from build123d import *

# Parameters (mm, degrees)
F0_W     = 25
F0_H     = 20
F1_DEPTH = 1
F3_DEPTH = 8


with BuildPart() as f1:
    # F0 (on Top) → F1 (new body)
    with BuildSketch(Plane.XY):
        Rectangle(F0_W, F0_H)
    extrude(amount=F1_DEPTH)

    # F2 (on Front) → F3 (join, symmetric)
    with BuildSketch(Plane.XZ):
        with BuildLine():
            Line((8.940514, 3.397746), (1.101284, 7.244365))
            ThreePointArc((1.101284, 7.244365), (0, 7.5), (-1.101284, 7.244365))
            Line((-1.101284, 7.244365), (-8.940514, 3.397746))
            ThreePointArc((-8.940514, 3.397746), (-9.348679, 3.028908), (-9.5, 2.5))
            Line((-9.5, 2.5), (-9.5, 0.999067))
            Line((-9.5, 0.999067), (9.5, 0.999067))
            Line((9.5, 0.999067), (9.5, 2.5))
            ThreePointArc((9.5, 2.5), (9.348679, 3.028908), (8.940514, 3.397746))
        make_face()
    extrude(amount=F3_DEPTH, both=True)


solid = f1.part
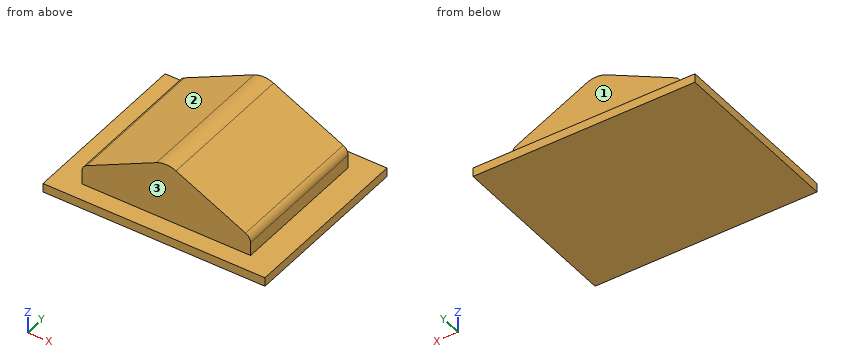
Could you check a few things on this model? Use its own coordinates, in mm. Face numbers are marked on the shaded views. A direction names the side the tool comes from. Give positions to 0.01 mm unless a question says otherwise; leave off trailing zeros. Order: outer loops, then holes, each group sorted by start corner. A loop starts at its lowest first (then second) coordinate and runs counter-clockwise, first axis right, second up. Notation, with made-up numbers: (55.5, -21) - (111.5, -21) arc R13 ccw to (111.5, -12) - close; hole circle Ø6 at (-35.75, 29). An arc over 180 degrees is marked (long way). Return JSON: item names as keys, results as strings. Group by question number.
Q1. Will these pins go through, and if not, where does the flat tip stop? pin 1 Ø0.8 at (y, z) = (-0.5, 1.5) entering from -X; pin 2 Ø0.8 at (y, z) = (-2.5, 1.5) entering from +X; pin 3 Ø6 at (x, y) = (-4.5, 2) entering from +Z.
Q2. Suppose I cut it at B-B, the plane x = -7.75. Please give me the cut outline in (y, z).
Q3. Suppose I cut it at D-D, the plane x = 3.75. Please give me the cut outline in (y, z).
Q4. Suppose I cut it at A-A, the plane y = -0.5. Please give me the cut outline in (x, z), and give its area (3 significant figures).
Q5. Suppose I cut it at C-C, the plane z = 1.5. Please give me the cut outline in (x, y).
Q6. Which directions (+Z, -Z, +X, -X, +Y, -Y) give clear straight access to the entire face, cutting with the end or side of a thin tool? Please do the marked faces 1, 2 and 3.
Q7. Please list where these lines run through material, in increasing order: line 1 along Y through (x, z) = (4.5, 5.25); line 2 along X through (y, z) = (5.5, 1.5); line 3 along Z through (x, y) = (4.25, -7). Write a range as [from, to].
Resolved:
{
 "1": {"pin 1": "stops at x = -9.5", "pin 2": "stops at x = 9.5", "pin 3": "stops at z = 7.05"},
 "2": {"outline": "(-10, 0) - (10, 0) - (10, 1) - (8, 1) - (8, 3.98) - (-8, 3.98) - (-8, 1) - (-10, 1) - close"},
 "3": {"outline": "(-10, 0) - (10, 0) - (10, 1) - (8, 1) - (8, 5.94) - (-8, 5.94) - (-8, 1) - (-10, 1) - close"},
 "4": {"outline": "(-12.5, 0) - (12.5, 0) - (12.5, 1) - (9.5, 1) - (9.5, 2.5) arc R1 ccw to (8.94, 3.4) - (1.1, 7.24) arc R2.5 ccw to (-1.1, 7.24) - (-8.94, 3.4) arc R1 ccw to (-9.5, 2.5) - (-9.5, 1) - (-12.5, 1) - close", "area": "109 mm2"},
 "5": {"outline": "(-9.5, -8) - (9.5, -8) - (9.5, 8) - (-9.5, 8) - close"},
 "6": {"face 1": "+Z, +X, -X, +Y", "face 2": "+Z, -X, +Y, -Y", "face 3": "+Z, +X, -X, -Y"},
 "7": {"line 1": "y = [-8, 8]", "line 2": "x = [-9.5, 9.5]", "line 3": "z = [0, 5.7]"}
}
